Source: CAD feature listing. Evaluate the final solid. Frame: model axes, mm. A direction names the side the tool comes from. Coordinates: 2 decimals unless noted, no trailing zeros. Loops run counter-clockwise (first coordinate to the right, second up) from the corner with the lowest first, then second, coordinate; pieces in that order, holes last. Notation, with made-up numbers: M 78,-0.75 L 114,-0.75 A16 ccw 114,19.25 Z; hole C 47,81 d6. An arc over 180 degrees is marked long. One line per question, with ' | ' between items. Start each with the question number.
1. Access query for faces 4 (the cylindrical face through (-14.4, 19.43, 16.55)), 5 (the cylindrical face through (-19.522, -23.472, 14.466)), 6 (the flat face through (0, -22, 13)). Directions: +Z, -Z, +X, -X, +Y, -Y. A direction counts if a zero-diameter tool reaches every point of the face in a straight line with its end or side. Return the directions, or none.
2. Mould query, pull axis Z, two halves, no side actions, for faces 1 (the cylindrical face through (-18, 21, 12)), 2 (the cylindrical face through (23.472, -19.522, 14.466)), 3 (the flat face through (-20, -20, 15)). Classes: pulls with the +Z half, pulls with the -Z half, needs draft (parallel to the pull), parting line crosses it, or undercut.
3. Ray query, probe 1 along X at (y, z) = (9.5, 16.75); probe 2 along X at (y, z) = (18, 16.75); probe 3 along Z at (x, y) = (-21, 23.3). Return the intervals inside material, ascending.
4. Section query D-D, the plane z = 10.5. Output: boundary loops of the cut face in (x, y), and give its area (3 significant figures).
5. Section query B-B, the plane x = 1. Output: boundary loops of the cut face in (y, z), and give its area (3 significant figures).
6. Pin query (flat end, axial travel): P1, Ø1.5, axis at x = 13, y = 20, coming from the -Z side; P2, Ø1.5, axis at x = 20, y = -20, coming from the +Z side; P3, Ø1.2, axis at y = -20.5, z = 14, coming from the +X side; P4, Ø4, axis at x = 21, z = 14, coming from the -Y side. Return the tip coordinate at first contact, or that it passes through.
7. Section query A-A, the plane z = 4.25. Output: boundary loops of the cut face in (x, y), and give its area (3 significant figures).
```python
from build123d import *

# Parameters (mm, degrees)
SKETCH_W        = 50
SKETCH_H        = 50
PAD_DEPTH       = 20
POCKET_DEPTH    = 20.001
POCKET001_DEPTH = 50.001
POCKET002_DEPTH = 50.001
SKETCH004_R     = 1.55
POCKET003_DEPTH = 4
SKETCH006_R     = 1.55
POCKET005_DEPTH = 4
SKETCH007_R     = 1.55
POCKET006_DEPTH = 4
SKETCH008_R     = 1.55
POCKET007_DEPTH = 4
SKETCH009_R     = 1.55
POCKET008_DEPTH = 5


with BuildPart() as part:
    # Sketch → Pad (new body)
    with BuildSketch(Plane.XY):
        Rectangle(SKETCH_W, SKETCH_H)
    extrude(amount=PAD_DEPTH)

    # Sketch001 (on Face6 of Pad) → Pocket (cut, through all)
    with BuildSketch(Plane.XY.offset(20)):
        with BuildLine():
            Line((-18, 15), (-17, 15))
            ThreePointArc((-17, 15), (-15.585786, 15.585786), (-15, 17))
            Line((-15, 17), (-15, 18))
            ThreePointArc((-13, 20), (-14.414214, 19.414214), (-15, 18))
            Line((-13, 20), (13, 20))
            ThreePointArc((15, 18), (14.414214, 19.414214), (13, 20))
            Line((15, 18), (15, 17))
            ThreePointArc((15, 17), (15.585786, 15.585786), (17, 15))
            Line((17, 15), (18, 15))
            ThreePointArc((20, 13), (19.414214, 14.414214), (18, 15))
            Line((20, 13), (20, -13))
            ThreePointArc((18, -15), (19.414214, -14.414214), (20, -13))
            Line((18, -15), (17, -15))
            ThreePointArc((17, -15), (15.585786, -15.585786), (15, -17))
            Line((15, -17), (15, -18))
            ThreePointArc((13, -20), (14.414214, -19.414214), (15, -18))
            Line((13, -20), (-13, -20))
            ThreePointArc((-15, -18), (-14.414214, -19.414214), (-13, -20))
            Line((-15, -18), (-15, -17))
            ThreePointArc((-15, -17), (-15.585786, -15.585786), (-17, -15))
            Line((-17, -15), (-18, -15))
            ThreePointArc((-20, -13), (-19.414214, -14.414214), (-18, -15))
            Line((-20, -13), (-20, 13))
            ThreePointArc((-18, 15), (-19.414214, 14.414214), (-20, 13))
        make_face()
    extrude(amount=-POCKET_DEPTH, mode=Mode.SUBTRACT)

    # Sketch002 (on Face3 of Pocket) → Pocket001 (cut, through all)
    with BuildSketch(Plane.YZ.offset(25)):
        with BuildLine():
            Line((-15, 13), (15, 13))
            ThreePointArc((20, 8), (18.535534, 11.535534), (15, 13))
            Line((20, 8), (20, 0))
            Line((20, 0), (-20, 0))
            Line((-20, 0), (-20, 8))
            ThreePointArc((-15, 13), (-18.535534, 11.535534), (-20, 8))
        make_face()
    extrude(amount=-POCKET001_DEPTH, mode=Mode.SUBTRACT)

    # Sketch003 (on Face6 of Pocket) → Pocket002 (cut, through all)
    with BuildSketch(Plane.XZ.offset(25)):
        with BuildLine():
            Line((-15, 13), (15, 13))
            ThreePointArc((20, 8), (18.535534, 11.535534), (15, 13))
            Line((20, 8), (20, 0))
            Line((20, 0), (-20, 0))
            Line((-20, 0), (-20, 8))
            ThreePointArc((-15, 13), (-18.535534, 11.535534), (-20, 8))
        make_face()
    extrude(amount=-POCKET002_DEPTH, mode=Mode.SUBTRACT)

    # Sketch004 (on Face11 of Pocket002) → Pocket003 (cut)
    with BuildSketch(Plane(origin=(-25, 0, 0), x_dir=(0, -1, 0), z_dir=(-1, 0, 0))):
        with Locations((-21, 14)):
            Circle(SKETCH004_R)
        with Locations((21, 14)):
            Circle(SKETCH004_R)
    extrude(amount=-POCKET003_DEPTH, mode=Mode.SUBTRACT)

    # Sketch006 → Pocket005 (cut)
    with BuildSketch(Plane.YZ.offset(25)):
        with Locations((-21, 14)):
            Circle(SKETCH006_R)
        with Locations((21, 14)):
            Circle(SKETCH006_R)
    extrude(amount=-POCKET005_DEPTH, mode=Mode.SUBTRACT)

    # Sketch007 (on Face1 of Pocket005) → Pocket006 (cut)
    with BuildSketch(Plane(origin=(0, 25, 0), x_dir=(-1, 0, 0), z_dir=(0, 1, 0))):
        with Locations((-21, 14)):
            Circle(SKETCH007_R)
        with Locations((21, 14)):
            Circle(SKETCH007_R)
    extrude(amount=-POCKET006_DEPTH, mode=Mode.SUBTRACT)

    # Sketch008 (on Face16 of Pocket006) → Pocket007 (cut)
    with BuildSketch(Plane.XZ.offset(25)):
        with Locations((-21, 14)):
            Circle(SKETCH008_R)
        with Locations((21, 14)):
            Circle(SKETCH008_R)
    extrude(amount=-POCKET007_DEPTH, mode=Mode.SUBTRACT)

    # Sketch009 (on Face5 of Pocket007) → Pocket008 (cut)
    with BuildSketch(Plane.XY.offset(20)):
        with Locations((-20, 20)):
            Circle(SKETCH009_R)
        with Locations((20, 20)):
            Circle(SKETCH009_R)
        with Locations((20, -20)):
            Circle(SKETCH009_R)
        with Locations((-20, -20)):
            Circle(SKETCH009_R)
    extrude(amount=-POCKET008_DEPTH, mode=Mode.SUBTRACT)


solid = part.part
```
Taken from the geometry:
1) face 4: +Z, -Z | face 5: -Y | face 6: -Z, +Y, -Y
2) face 1: pulls with the -Z half | face 2: undercut | face 3: pulls with the +Z half
3) probe 1: -25 to -20, 20 to 25 | probe 2: -25 to -15, 15 to 25 | probe 3: 0 to 12.45, 15.55 to 20
4) outline: M -25,-25 L -19.33,-25 L -19.33,-19.33 L -25,-19.33 Z; M -25,19.33 L -19.33,19.33 L -19.33,25 L -25,25 Z; M 19.33,-25 L 25,-25 L 25,-19.33 L 19.33,-19.33 Z; M 19.33,19.33 L 25,19.33 L 25,25 L 19.33,25 Z | area: 129 mm^2
5) outline: M -25,13 L -20,13 L -20,20 L -25,20 Z; M 20,13 L 25,13 L 25,20 L 20,20 Z | area: 70.0 mm^2
6) P1: z = 13 | P2: z = 15 | P3: x = 21 | P4: y = -25
7) outline: M -25,-25 L -20,-25 L -20,-20 L -25,-20 Z; M -25,20 L -20,20 L -20,25 L -25,25 Z; M 20,-25 L 25,-25 L 25,-20 L 20,-20 Z; M 20,20 L 25,20 L 25,25 L 20,25 Z | area: 100 mm^2
